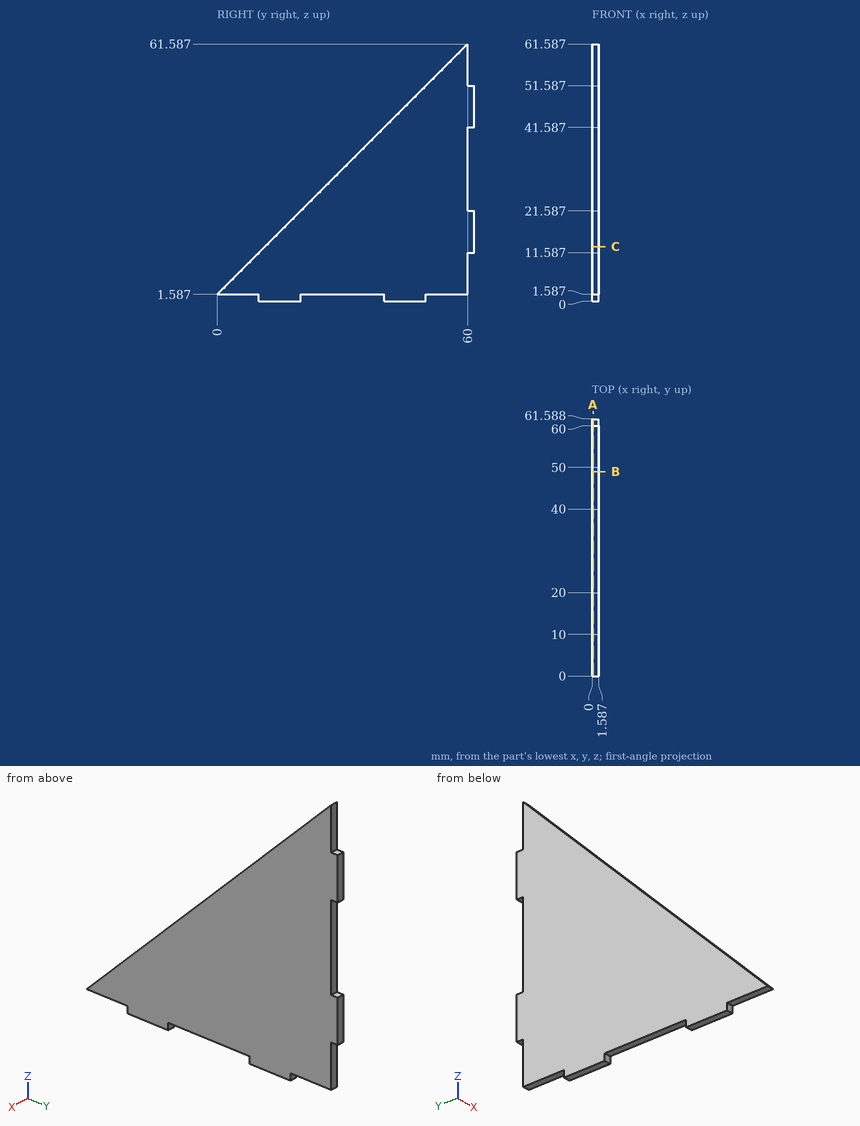
Source: three-view drawing plus pictorial views. Frame: mm from the lowest corner of the part. Round coordinates to 2 decimals unless told otherwise and drop trailing zeros. Loops run counter-clockwise (first coordinate to the right, second up) from the corner with the lowest first, then second, coordinate; pieces in that order, holes last.
1. Section query B-B on y = 49. Output: boundary loops of the cut face in (x, z).
2. Ray query, L1, parallel to Z at x = 0.5, y = 53.5 (1 decimal); L2, parallel to Z at x = 0.8, y = 8.5 (1 decimal); L3, parallel to Y at x = 0.8, z = 31 (1 decimal). Return the intervals inside material, ascending.
3. Contact query for flat-ended pins moving along their axis: pin 1 (0.8 mm diameter, centred on x = 0.5, z = 1, fed in from +Y); pin 2 (0.8 mm diameter, centred on x = 1, z = 57.5, fed in from +Y); pin 3 (0.8 mm diameter, centred on x = 0.5, y = 61, fed in from -Z). Output: stop coordinate, or through.
4. Section query C-C on z = 13. Output: boundary loops of the cut face in (x, y).
5. Section query A-A on x = 0.25. Output: boundary loops of the cut face in (y, z), and give its area (3 significant figures).
Answers below:
1. outline: (0, 0) - (1.59, 0) - (1.59, 50.59) - (0, 50.59) - close
2. L1: z = 1.6 to 55.1
2. L2: z = 1.6 to 10.1
2. L3: y = 29.4 to 60
3. pin 1: stops at y = 50
3. pin 2: stops at y = 60
3. pin 3: stops at z = 11.59
4. outline: (0, 11.41) - (1.59, 11.41) - (1.59, 61.59) - (0, 61.59) - close
5. outline: (0, 1.59) - (10, 1.59) - (10, 0) - (20, 0) - (20, 1.59) - (40, 1.59) - (40, 0) - (50, 0) - (50, 1.59) - (60, 1.59) - (60, 11.59) - (61.59, 11.59) - (61.59, 21.59) - (60, 21.59) - (60, 41.59) - (61.59, 41.59) - (61.59, 51.59) - (60, 51.59) - (60, 61.59) - close
5. area: 1,860 mm2
